```python
from build123d import *

# Parameters (mm, degrees)
SKETCH1_W           = 44
SKETCH1_H           = 25
BOSS_EXTRUDE1_DEPTH = 1.524
CHAMFER1_SIZE       = 0.25


with BuildPart() as part:
    # Sketch1 → Boss-Extrude1 (new body)
    with BuildSketch(Plane(origin=(0, 0, 0), x_dir=(1, 0, 0), z_dir=(0, 1, 0))):
        Rectangle(SKETCH1_W, SKETCH1_H)
        Polygon((-9.4996, 4.939226775), (-7, 4.939226775), (-7, 7), (7, 7), (7, 4.939226775), (9.4996, 4.939226775), (9.4996, 5.752026775), (16.1544, 5.752026775), (16.1544, 2.286), (17.174185585, 2.286), (17.174185585, -0.508), (16.1544, -0.508), (16.1544, -6.541573225), (13.462, -6.541573225), (13.462, -7.709973225), (10.414, -7.709973225), (10.414, -6.541573225), (9.4996, -6.541573225), (9.4996, -5.754173225), (7, -5.754173225), (7, -7), (-7, -7), (-7, -5.754173225), (-9.4996, -5.754173225), (-9.4996, -6.541573225), (-10.414, -6.541573225), (-10.414, -7.709973225), (-13.462, -7.709973225), (-13.462, -6.541573225), (-16.1544, -6.541573225), (-16.1544, -0.508), (-17.174185585, -0.508), (-17.174185585, 2.286), (-16.1544, 2.286), (-16.1544, 5.752026775), (-9.4996, 5.752026775), align=None, mode=Mode.SUBTRACT)
    extrude(amount=BOSS_EXTRUDE1_DEPTH)

    # Chamfer1
    chamfer1_edges = [part.edges().sort_by_distance(p)[0] for p in [
        (7, 0, -5.969613387),
        (0, 0, -7),
        (-7, 0, -5.969613387),
        (-8.2498, 0, -4.939226775),
        (-9.4996, 0, -5.345626775),
        (-12.827, 0, -5.752026775),
        (-16.1544, 0, -4.019013387),
        (-16.664292792, 0, -2.286),
        (-17.174185585, 0, -0.889),
        (-16.664292792, 0, 0.508),
        (-16.1544, 0, 3.524786613),
        (-14.8082, 0, 6.541573225),
        (-13.462, 0, 7.125773225),
        (-11.938, 0, 7.709973225),
        (-10.414, 0, 7.125773225),
        (-9.9568, 0, 6.541573225),
        (-9.4996, 0, 6.147873225),
        (-8.2498, 0, 5.754173225),
        (-7, 0, 6.377086613),
        (0, 0, 7),
        (7, 0, 6.377086613),
        (8.2498, 0, 5.754173225),
        (9.4996, 0, 6.147873225),
        (9.9568, 0, 6.541573225),
        (10.414, 0, 7.125773225),
        (11.938, 0, 7.709973225),
        (13.462, 0, 7.125773225),
        (14.8082, 0, 6.541573225),
        (16.1544, 0, 3.524786613),
        (16.664292792, 0, 0.508),
        (17.174185585, 0, -0.889),
        (16.664292792, 0, -2.286),
        (16.1544, 0, -4.019013387),
        (12.827, 0, -5.752026775),
        (9.4996, 0, -5.345626775),
        (8.2498, 0, -4.939226775),
        (0, 0, 12.5),
        (-22, 0, 0),
        (0, 0, -12.5),
        (22, 0, 0),
    ]]
    chamfer(chamfer1_edges, length=CHAMFER1_SIZE)


solid = part.part
```
Input: part model. Units: mm. Frame: model coordinates. A direction names the side the tool comes from. Round coordinates to 2 decimals unless told otherwise and drop trailing zeros. Loops run counter-clockwise (first coordinate to the right, second up) from the corner with the lowest first, then second, coordinate; pieces in that order, holes last.
1) Pull-direction query (X, two-part tool) for faces 1 (the flat face through (-22, 1, 0)), 2 (the flat face through (0, 1, 7)), 3 (the flat face through (0, 0, -8)); classes: released by +X, released by -X, zero draft, split by the parting line, or undercut.
Ans:
face 1: released by -X
face 2: undercut
face 3: zero draft
2) Section query B-B on z = -1.75. Return the cut outline in (x, y), plus the area to 3 significant figures.
Ans:
outline: (-22, 0.25) - (-21.75, 0) - (-17.42, 0) - (-17.17, 0.25) - (-17.17, 1.52) - (-22, 1.52) - close; (17.17, 0.25) - (17.42, 0) - (21.75, 0) - (22, 0.25) - (22, 1.52) - (17.17, 1.52) - close
area: 14.6 mm2
3) Set-up query: faces 4 (the flat face through (0, 1, 12.5)), 5 (the flat face through (-16.154, 1, 4)). Return all of +Z, -Z, +X, -X, +Y, -Y with unobstructed straight access to the full face (end or side cutting, diameter ignored); none if empty.
Ans:
face 4: +Z, +X, -X, +Y, -Y
face 5: +Y, -Y
4) Section query A-A on x = 11.5. Return the cut outline in (y, z), plus the area to 3 significant figures.
Ans:
outline: (0, -12.25) - (0.25, -12.5) - (1.52, -12.5) - (1.52, -5.75) - (0.25, -5.75) - (0, -6) - close; (0, 7.96) - (0.25, 7.71) - (1.52, 7.71) - (1.52, 12.5) - (0.25, 12.5) - (0, 12.25) - close
area: 17.5 mm2
5) Material intervals for line 1 (Z direction, x = 2, y = 0.35); line 2 (Z direction, x = -16.5, y = 0.35); line 3 (X direction, y = 0.5, z = 1.25), sorted ascending.
Ans:
line 1: z = -12.5 to -7, 7 to 12.5
line 2: z = -12.5 to -2.29, 0.51 to 12.5
line 3: x = -22 to -16.15, 16.15 to 22
